```python
from build123d import *

# Parameters (mm, degrees)
SKETCH_1_R          = 1.6
EXTRUDE_1_DEPTH     = 2
SKETCH_2_R          = 1.05
CUT_EXTRUDE_1_DEPTH = 10


with BuildPart() as part:
    # 草图1 → 凸台-拉伸1 (new body)
    with BuildSketch(Plane.XY):
        with BuildLine():
            Line((-10.162831426, 3), (10.162831426, 3))
            ThreePointArc((10.162831426, 3), (11.749775558, 5.55230577), (13.5, 7.995535358))
            Line((13.5, 7.995535358), (13.5, 26.5))
            Line((13.5, 26.5), (37.5, 26.5))
            Line((37.5, 26.5), (37.5, 20.096757974))
            ThreePointArc((37.5, 20.096757974), (22.049805692, 11.349428036), (11.594271261, -3))
            Line((11.594271261, -3), (-11.594271261, -3))
            ThreePointArc((-11.594271261, -3), (-22.049805692, 11.349428036), (-37.5, 20.096757974))
            Line((-37.5, 20.096757974), (-37.5, 26.5))
            Line((-37.5, 26.5), (-13.5, 26.5))
            Line((-13.5, 26.5), (-13.5, 7.995535358))
            ThreePointArc((-13.5, 7.995535358), (-11.749775558, 5.55230577), (-10.162831426, 3))
        make_face()
        Circle(SKETCH_1_R, mode=Mode.SUBTRACT)
    extrude(amount=EXTRUDE_1_DEPTH)

    # 草图2 → 切除-拉伸1 (cut)
    with BuildSketch(Plane.XY.offset(2)):
        with Locations((-32.5, 24.5)):
            Circle(SKETCH_2_R)
        with Locations((-16, 24.5)):
            Circle(SKETCH_2_R)
        with Locations((16, 24.5)):
            Circle(SKETCH_2_R)
        with Locations((32.5, 24.5)):
            Circle(SKETCH_2_R)
    extrude(amount=-CUT_EXTRUDE_1_DEPTH, mode=Mode.SUBTRACT)


solid = part.part
```
CAD build for the part. Positions are in the model's coordinates, mm. A direction names the side the tool comes from. Round coordinates to 2 decimals unless told otherwise and drop trailing zeros. Loops run counter-clockwise (first coordinate to the right, second up) from the corner with the lowest first, then second, coordinate; pieces in that order, holes last. Notation, with made-up numbers: (-2, 62) - (7, 62) arc R22 ccw to (7, 76) - close; hole circle Ø5 at (73.5, -19). An arc over 180 degrees is marked (long way). Return JSON: item names as keys, results as strings. Group by question number.
Q1. Band-saw the part on D-D on x = -9.5. Give the cut face in (y, z), plus the area to 3 significant figures.
Q2. Band-saw the part on C-C on z = 0.9. Give the cut face in (x, y), plus the area to 3 significant figures.
Q3. Two-plate mould, pull along Y, no slides. Class faces 1 (the face through (25, 26.5, 1)), 2 (the face through (-21.86, 11.18, 0.99)), 3 (the face through (0, 2, 2)), 4 (the face through (-32.015, 23.568, 1.014)): +Y half, -Y half, draft (parallel to the pull), parting line (faces both ways), or undercut.
Q4. Tool access for faces 5 (the face through (37.5, 23, 1)), 6 (the face through (0, 3, 1)): list every direction of +Z, -Z, +X, -X, +Y, -Y with a clear straight run to the whole face (end or side of a thin tool).
Q5. Flat gauge pin, fed straight in: pin 1 Ø0.6 at (x, z) = (2.5, 1) entering from +Y. Where does the tip first touch, or does it go through?
Q6. Band-saw the part on A-A on x = 0. Give the cut face in (y, z).
Q7. Band-saw the part on B-B on y = 22.75. Give the cut face in (x, z), plus the area to 3 significant figures.
Q8. Drill centre lines: line 1 along X through (y, z) = (20.5, 1.25); line 2 along X through (y, z) = (18.25, 0.45); line 3 along Y through (x, z) = (16, 0.5). Where is each one in solid material? Low to high. Write a range as [from, to].
Solutions:
{
 "1": {"outline": "(-3, 0) - (3, 0) - (3, 2) - (-3, 2) - close", "area": "12.0 mm^2"},
 "2": {"outline": "(-37.5, 20.1) arc R42 cw to (-11.59, -3) - (11.59, -3) arc R42 cw to (37.5, 20.1) - (37.5, 26.5) - (13.5, 26.5) - (13.5, 8) arc R46 ccw to (10.16, 3) - (-10.16, 3) arc R46 ccw to (-13.5, 8) - (-13.5, 26.5) - (-37.5, 26.5) - close; hole circle Ø2.1 at (-32.5, 24.5); hole circle Ø2.1 at (-16, 24.5); hole circle Ø3.2 at (0, 0); hole circle Ø2.1 at (16, 24.5); hole circle Ø2.1 at (32.5, 24.5)", "area": "800 mm^2"},
 "3": {"face 1": "+Y half", "face 2": "-Y half", "face 3": "draft", "face 4": "undercut"},
 "4": {"face 5": "+Z, -Z, +X, +Y, -Y", "face 6": "+Z, -Z, +Y"},
 "5": {"pin 1": "stops at y = 3"},
 "6": {"outline": "(-3, 0) - (-1.6, 0) - (-1.6, 2) - (-3, 2) - close; (1.6, 0) - (3, 0) - (3, 2) - (1.6, 2) - close"},
 "7": {"outline": "(-37.5, 0) - (-13.5, 0) - (-13.5, 2) - (-37.5, 2) - close; (13.5, 0) - (37.5, 0) - (37.5, 2) - (13.5, 2) - close", "area": "96.0 mm^2"},
 "8": {"line 1": "x = [-37.5, -13.5], [13.5, 37.5]", "line 2": "x = [-32.65, -13.5], [13.5, 32.65]", "line 3": "y = [4.66, 23.45], [25.55, 26.5]"}
}
